```python
from build123d import *

# Parameters (mm, degrees)
BASPROSKE_W        = 15
BASPROSKE_H        = 24.75
TOOTHCUT_DEPTH     = 39.080506824
TEETHCUTS_COUNT    = 20
BORSKE_R           = 6
BORE_DEPTH         = 50.0000508
SKETCH1_R          = 6
CUT_EXTRUDE1_DEPTH = 7
CUT_EXTRUDE2_DEPTH = 7


with BuildPart() as part:
    # BasProSke → Base-Revolve (revolve)
    with BuildSketch(Plane(origin=(0, 0, 0), x_dir=(1, 0, 0), z_dir=(0, 1, 0)), mode=Mode.PRIVATE) as base_revolve_sk:
        with Locations((7.5, 12.375)):
            Rectangle(BASPROSKE_W, BASPROSKE_H)
    revolve(base_revolve_sk.sketch.rotate(Axis((-10, 0, 0), (1, 0, 0)), 180), axis=Axis((-10, 0, 0), (1, 0, 0)))

    # TooCutSke → ToothCut (cut, through all)
    with BuildSketch(Plane(origin=(0, 0, 0), x_dir=(0, 0, -1), z_dir=(1, 0, 0))):
        with BuildLine():
            ThreePointArc((1.111948432, 19.655071939), (0, 19.6865), (-1.111948432, 19.655071939))
            ThreePointArc((-1.111948432, 19.655071939), (-1.832349961, 22.271720111), (-3.300041734, 24.55463642))
            ThreePointArc((-3.300041734, 24.55463642), (0, 24.7754), (3.300041734, 24.55463642))
            ThreePointArc((3.300041734, 24.55463642), (1.832349961, 22.271720111), (1.111948432, 19.655071939))
        make_face()
    toothcut = extrude(amount=TOOTHCUT_DEPTH, mode=Mode.SUBTRACT)

    # TeethCuts: ToothCut ×20 about axis
    teethcuts_axis = Axis((0, 0, 0), (1, 0, 0))
    for i in range(1, TEETHCUTS_COUNT):
        add(toothcut.rotate(teethcuts_axis, i * 360 / TEETHCUTS_COUNT), mode=Mode.SUBTRACT)

    # BorSke → Bore (cut, symmetric)
    with BuildSketch(Plane(origin=(0, 0, 0), x_dir=(0, 0, -1), z_dir=(1, 0, 0))):
        with Locations(Location((0, 0, 0), (0, 0, 180))):
            Circle(BORSKE_R)
    extrude(amount=BORE_DEPTH, both=True, mode=Mode.SUBTRACT)

    # Sketch1 → Cut-Extrude1 (cut)
    with BuildSketch(Plane(origin=(15, 0, 0), x_dir=(0, 0, -1), z_dir=(1, 0, 0))):
        with BuildLine():
            ThreePointArc((6, 0), (4.255305349, 4.229938107), (0.035874537, 5.999892751))
            Line((0.035874537, 5.999892751), (5.064141431, -3.217836473))
            ThreePointArc((5.064141431, -3.217836473), (5.761286687, -1.675582199), (6, 0))
        make_face()
        with BuildLine():
            Line((5.064141431, -3.217836473), (0.035874537, 5.999892751))
            ThreePointArc((0.035874537, 5.999892751), (-5.267273842, -2.873295368), (5.064141431, -3.217836473))
        make_face()
        with Locations(Location((0, 0, 0), (0, 0, 89.657421369))):
            Circle(SKETCH1_R)
        Polygon((0.035874537, 5.999892751), (5.064141431, -3.217836473), (14.281870655, 1.810430421), (9.25360376, 11.028159645), align=None)
    extrude(amount=-CUT_EXTRUDE1_DEPTH, mode=Mode.SUBTRACT)

    # Sketch2 → Cut-Extrude2 (cut)
    with BuildSketch(Plane.ZY):
        Polygon((13.03803352, -4.691447745), (10.581929687, 8.945544371), (-2.456103832, 13.636992116), (-13.03803352, 4.691447745), (-10.581929687, -8.945544371), (2.456103832, -13.636992116), align=None)
        Polygon((13.636992116, 2.456103832), (4.691447745, 13.03803352), (-8.945544371, 10.581929687), (-13.636992116, -2.456103832), (-4.691447745, -13.03803352), (8.945544371, -10.581929687), align=None)
        Polygon((-13.636992116, -2.456103832), (-11.240040726, -5.291523347), (-12.379922481, 1.03742672), align=None)
        Polygon((-10.581929687, -8.945544371), (-7.088399135, -10.202614006), (-11.240040726, -5.291523347), align=None)
        Polygon((-4.691447745, -13.03803352), (-1.03742672, -12.379922481), (-7.088399135, -10.202614006), align=None)
        Polygon((2.456103832, -13.636992116), (5.291523347, -11.240040726), (-1.03742672, -12.379922481), align=None)
        Polygon((8.945544371, -10.581929687), (10.202614006, -7.088399135), (5.291523347, -11.240040726), align=None)
        Polygon((10.202614006, -7.088399135), (13.03803352, -4.691447745), (12.379922481, -1.03742672), align=None)
        Polygon((7.088399135, 10.202614006), (11.240040726, 5.291523347), (10.581929687, 8.945544371), align=None)
        Polygon((11.240040726, 5.291523347), (12.379922481, -1.03742672), (13.636992116, 2.456103832), align=None)
        Polygon((1.03742672, 12.379922481), (7.088399135, 10.202614006), (4.691447745, 13.03803352), align=None)
        Polygon((-5.291523347, 11.240040726), (1.03742672, 12.379922481), (-2.456103832, 13.636992116), align=None)
        Polygon((-10.202614006, 7.088399135), (-5.291523347, 11.240040726), (-8.945544371, 10.581929687), align=None)
        Polygon((-12.379922481, 1.03742672), (-10.202614006, 7.088399135), (-13.03803352, 4.691447745), align=None)
    extrude(amount=-CUT_EXTRUDE2_DEPTH, mode=Mode.SUBTRACT)


solid = part.part
```
Check sheet for the modelled part. Datum: model origin and axes. Units: mm. A direction names the side the tool comes from. Give positions to 0.01 mm unless a question says otherwise; leave off trailing zeros. Write each loop counter-clockwise with the first axis right and the second up, starting at its lowest first coordinate (ties: lowest second). Pieces come first, ordered by that corner, then holes. Notation, with made-up numbers: (-20.5, 0) - (17.5, 0) arc R26 ccw to (17.5, 29) - close; hole circle Ø3 at (75, -28.5). An arc over 180 degrees is marked (long way). Answer as a JSON object with one key per item and string values. Group by question number.
1) Thickness scan on probe 1 along Y at (x, z) = (10, 0); probe 2 along Y at (x, z) = (11.5, 16.5); probe 3 along Z at (x, y) = (6.5, 20.5). Record the ranges inside material, lowest first. Write a range as from..to.
2) Access from +Z, -Z, +X, -X, +Y, -Y to the whole of each face (thin tool, end or side, straight path). Record for faces 1 (the face through (7.4, -22.2, -1.8)), 2 (the face through (3.451, -8.86, 9.565)), 3 (the face through (7.395, 5.137, -21.77)), 4 (the face through (7.605, 22.056, 11.229)), 5 (the face through (11.549, 6.355, -11.803)).
3) Sectioned sample at B-B (y = 0). Record the cut outline in (x, z), then the cut area to 3 significant figures.
4) Release check for a two-part mould opening along Z. For faces 6 (the face through (3.451, -9.565, -8.86)), 7 (the face through (7.605, 24.444, -3.88)), 8 (the face through (7.395, 21.77, 5.137)), 9 (the face through (7.605, 3.88, 24.444)) record: pulls with the +Z half, pulls with the -Z half, needs draft (parallel to the pull), parting line crosses it, or undercut.
5) Depth check by flat-ended pin: P1, Ø8, axis at y = -3, z = 4, coming from the -X side; P2, Ø1, axis at y = 7.5, z = -7.5, coming from the +X side; P3, Ø5, axis at x = 3, z = -12.5, coming from the -Y side; P4, Ø11, axis at y = 0, z = 0, coming from the +X side. Enter the tip coordinate at first touch or a pass-through.
6) Sectioned sample at A-A (z = -8). Record the cut outline in (x, y), then the cut area to 3 significant figures.
Geometry results:
{
 "1": {"probe 1": "y = -19.69..-6, 6..19.69", "probe 2": "y = -17.77..-13.88, -10.74..10.74, 13.88..17.77", "probe 3": "z = -11.79..-8.52, -5.19..-1.25, 1.25..5.19, 8.52..11.79"},
 "2": {"face 1": "+X, -X, -Y", "face 2": "-X", "face 3": "+X, -X", "face 4": "+Z, +X, -X, +Y", "face 5": "+X"},
 "3": {"outline": "(0, -19.69) - (15, -19.69) - (15, -10.96) - (8, -10.96) - (8, -6) - (7, -6) - (7, -12.75) - (0, -12.75) - close; (0, 12.75) - (7, 12.75) - (7, 6) - (15, 6) - (15, 19.69) - (0, 19.69) - close", "area": "281 mm^2"},
 "4": {"face 6": "undercut", "face 7": "pulls with the -Z half", "face 8": "undercut", "face 9": "pulls with the +Z half"},
 "5": {"P1": "stops at x = 7", "P2": "stops at x = 8", "P3": "stops at y = -22.32", "P4": "passes through"},
 "6": {"outline": "(0, -19.84) - (15, -19.84) - (15, -1.62) - (8, -1.62) - (8, 10.34) - (15, 10.34) - (15, 19.84) - (0, 19.84) - (0, 10.75) - (7, 10.75) - (7, -9.87) - (0, -9.87) - close", "area": "367 mm^2"}
}
